The model under review builds one solid part; all positions refer to its coordinate system, in mm. A direction names the side the tool comes from. Round coordinates to 2 decimals unless told otherwise and drop trailing zeros. Order: outer loops, then holes, each group sorted by start corner. A loop starts at its lowest first (then second) coordinate and runs counter-clockwise, first axis right, second up. Notation, with made-up numbers: M -16.75,4.25 L 17.25,4.25 A21 ccw 17.25,22.25 Z; hole C -17,-12.75 d7. An arc over 180 degrees is marked long. Use a Markdown table: item, result. Add a question column.
1. Consider section D-D on y = 54. State the section outline as (x, z) points, then the cut area to 3 significant figures.
2. Consider section B-B on z = 23. State the section outline as (x, y) points, then the cut area to 3 significant figures.
3. Insertion check: P1, Ø9.5, axis at x = -16.5, y = 43, coming from the -Z side; P2, Ø12, axis at x = 20, y = 50, coming from the +Z side; P3, Ø9.5, axis at x = 22.5, y = 24, coming from the +Z side. Each pin has a flat end and moves straight along its axis. Give the tip position at first contact, or say it passes through.
4. For faces 5 (the flat face through (-4.5, 1, 20)), 6 (the cylindrical face through (34, 5.4, 33.9)), 7 (the flat face through (-11, 46, -11)), 8 (the flat face through (11, 46, 11)), list the 3-axis set-ups (+Z, -Z, +X, -X, +Y, -Y) from which the entire face can be reached by the end or side of a thin tool; tool diameter is ignored.
5. Consider section A-A on y = 63. State the section outline as (x, z) points.
6. To check wall thickness, follow probe 1 along X at (y, z) = (7, -29); probe 2 along Z at (x, y) = (0, 74); probe 3 along Y at (x, z) = (-7, 6.5). State the ranges of each line that lie inside material, in increasing order.
7. The part is to be moulded in two halves that separate along Z. For faces 1 (the flat face through (0, 5, -36)), 2 (the flat face through (-20, 1, -4.5)), 3 (the flat face through (36, 5, 0)), 4 (the cylindrical face through (-11.99, 76.07, -0.53)), say which applies: +Z half, -Z half, draft (parallel to the pull), parting line (faces both ways), or undercut.
8. Consider section C-C on x = 21.5. State the section outline as (y, z) points.
from build123d import *

# Parameters (mm, degrees)
EXTRUDE_1_DEPTH              = 11
EXTRUDE_2_DEPTH              = 4.5
EXTRUDE_3_DEPTH              = 4.5
EXTRUDE_4_DEPTH              = 35
HOLE_WIZARD_M4_1_D           = 18
HOLE_WIZARD_M4_1_DEPTH       = 20
HOLE_WIZARD_M4_1_CBORE_D     = 24
HOLE_WIZARD_M4_1_CBORE_DEPTH = 10
HOLE_WIZARD_M4_1_TIP         = 5.407745571
SKETCH_14_R                  = 4
CUT_EXTRUDE_1_DEPTH          = 15
CUT_EXTRUDE_2_DEPTH          = 96.671312315
CUT_EXTRUDE_2_DEPTH_BACK     = 96.671312315
SKETCH_15_W                  = 9
SKETCH_15_H                  = 3
CUT_EXTRUDE_3_DEPTH          = 96.671312315
CUT_EXTRUDE_3_DEPTH_BACK     = 96.671312315
SKETCH_16_W                  = 9
SKETCH_16_H                  = 3


with BuildPart() as part:
    # 스케치1 → 보스-돌출1 (new body)
    with BuildSketch(Plane(origin=(0, 0, 0), x_dir=(1, 0, 0), z_dir=(0, 1, 0))):
        with BuildLine():
            Line((-29, 36), (29, 36))
            ThreePointArc((29, 36), (33.949747468, 33.949747468), (36, 29))
            Line((36, 29), (36, -29))
            ThreePointArc((36, -29), (33.949747468, -33.949747468), (29, -36))
            Line((29, -36), (-29, -36))
            ThreePointArc((-29, -36), (-33.949747468, -33.949747468), (-36, -29))
            Line((-36, -29), (-36, 29))
            ThreePointArc((-36, 29), (-33.949747468, 33.949747468), (-29, 36))
        make_face()
    extrude(amount=EXTRUDE_1_DEPTH)

    # 스케치2 → 보스-돌출2 (add, symmetric)
    with BuildSketch(Plane.XY):
        Polygon((-36, 11), (-13.651164073, 66.315309992), (13.651164073, 66.315309992), (36, 11), align=None)
    extrude(amount=EXTRUDE_2_DEPTH, both=True)

    # 스케치3 → 보스-돌출3 (add, symmetric)
    with BuildSketch(Plane(origin=(0, 0, 0), x_dir=(0, 0, -1), z_dir=(1, 0, 0))):
        Polygon((-36, 11), (-13.651164073, 66.315309992), (13.651164073, 66.315309992), (36, 11), align=None)
    extrude(amount=EXTRUDE_3_DEPTH, both=True)

    # 스케치4 → 보스-돌출4 (add)
    with BuildSketch(Plane(origin=(0, 81, 0), x_dir=(1, 0, 0), z_dir=(0, 1, 0))):
        with BuildLine():
            Line((-7.5, 17.5), (7.5, 17.5))
            ThreePointArc((7.5, 17.5), (14.571067812, 14.571067812), (17.5, 7.5))
            Line((17.5, 7.5), (17.5, -7.5))
            ThreePointArc((17.5, -7.5), (14.571067812, -14.571067812), (7.5, -17.5))
            Line((7.5, -17.5), (-7.5, -17.5))
            ThreePointArc((-7.5, -17.5), (-14.571067812, -14.571067812), (-17.5, -7.5))
            Line((-17.5, -7.5), (-17.5, 7.5))
            ThreePointArc((-17.5, 7.5), (-14.571067812, 14.571067812), (-7.5, 17.5))
        make_face()
    extrude(amount=-EXTRUDE_4_DEPTH)

    # M4 소켓 머리 캡 나사용 카운터보어1
    with Locations(Plane(origin=(0, 81, 0), x_dir=(1, 0, 0), z_dir=(0, 1, 0))):
        with Locations((0, 0)):
            CounterBoreHole(HOLE_WIZARD_M4_1_D / 2, HOLE_WIZARD_M4_1_CBORE_D / 2, HOLE_WIZARD_M4_1_CBORE_DEPTH, depth=HOLE_WIZARD_M4_1_DEPTH)
            with Locations((0, 0, -(HOLE_WIZARD_M4_1_DEPTH + HOLE_WIZARD_M4_1_TIP / 2))):  # 118° drill point
                Cone(0, HOLE_WIZARD_M4_1_D / 2, HOLE_WIZARD_M4_1_TIP, mode=Mode.SUBTRACT)

    # 스케치14 → 컷-돌출1 (cut)
    with BuildSketch(Plane.XZ):
        with Locations(Location((-29, 29, 0), (0, 0, 270))):
            Circle(SKETCH_14_R)
        with Locations(Location((29, 29, 0), (0, 0, 270))):
            Circle(SKETCH_14_R)
        with Locations(Location((-29, -29, 0), (0, 0, 270))):
            Circle(SKETCH_14_R)
        with Locations(Location((29, -29, 0), (0, 0, 270))):
            Circle(SKETCH_14_R)
    extrude(amount=-CUT_EXTRUDE_1_DEPTH, mode=Mode.SUBTRACT)

    # 스케치15 → 컷-돌출2 (cut, two sides: drawn at the far end of the back side and taken through both)
    with BuildSketch(Plane(origin=(0, 0, 0), x_dir=(0, 0, -1), z_dir=(1, 0, 0)).offset(-CUT_EXTRUDE_2_DEPTH_BACK)):
        with Locations((0, 1.5)):
            Rectangle(SKETCH_15_W, SKETCH_15_H)
    extrude(amount=CUT_EXTRUDE_2_DEPTH + CUT_EXTRUDE_2_DEPTH_BACK, mode=Mode.SUBTRACT)

    # 스케치16 → 컷-돌출3 (cut, two sides: drawn at the far end of the back side and taken through both)
    with BuildSketch(Plane.XY.offset(-CUT_EXTRUDE_3_DEPTH_BACK)):
        with Locations((0, 1.5)):
            Rectangle(SKETCH_16_W, SKETCH_16_H)
    extrude(amount=CUT_EXTRUDE_3_DEPTH + CUT_EXTRUDE_3_DEPTH_BACK, mode=Mode.SUBTRACT)


solid = part.part
Answer block:
| question | item | result |
|---|---|---|
| 1 | outline | M -18.63,-4.5 L -17.5,-4.5 L -17.5,-7.5 A10 ccw -7.5,-17.5 L -4.5,-17.5 L -4.5,-18.63 L 4.5,-18.63 L 4.5,-17.5 L 7.5,-17.5 A10 ccw 17.5,-7.5 L 17.5,-4.5 L 18.63,-4.5 L 18.63,4.5 L 17.5,4.5 L 17.5,7.5 A10 ccw 7.5,17.5 L 4.5,17.5 L 4.5,18.63 L -4.5,18.63 L -4.5,17.5 L -7.5,17.5 A10 ccw -17.5,7.5 L -17.5,4.5 L -18.63,4.5 Z |
| 1 | area | 1,180 mm^2 |
| 2 | outline | M -36,0 L -4.5,0 L -4.5,3 L 4.5,3 L 4.5,0 L 36,0 L 36,11 L 4.5,11 L 4.5,43.18 L -4.5,43.18 L -4.5,11 L -36,11 Z |
| 2 | area | 1,050 mm^2 |
| 3 | P1 | z = -15.97 |
| 3 | P2 | z = 15.1 |
| 3 | P3 | z = 4.5 |
| 4 | face 5 | +Z, -Z, -Y |
| 4 | face 6 | +Z, +X, +Y, -Y |
| 4 | face 7 | -Z, -X |
| 4 | face 8 | +Z, +X |
| 5 | outline | M -17.5,-7.5 A10 ccw -7.5,-17.5 L 7.5,-17.5 A10 ccw 17.5,-7.5 L 17.5,7.5 A10 ccw 7.5,17.5 L -7.5,17.5 A10 ccw -17.5,7.5 Z; hole C 0,0 d18 |
| 6 | probe 1 | -36 to -33, -25 to 25, 33 to 36 |
| 6 | probe 2 | -17.5 to -12, 12 to 17.5 |
| 6 | probe 3 | 0 to 11, 46 to 71 |
| 7 | face 1 | -Z half |
| 7 | face 2 | undercut |
| 7 | face 3 | draft |
| 7 | face 4 | undercut |
| 8 | outline | M 0,-36 L 11,-36 L 11,-4.5 L 46.89,-4.5 L 46.89,4.5 L 11,4.5 L 11,36 L 0,36 L 0,4.5 L 3,4.5 L 3,-4.5 L 0,-4.5 Z |
